The figure shows three views and two pictorial views of one solid part (mm, origin at its lowest corner). Answer the questions. A direction names the side the tool comes from. Give positions to 0.01 mm unless a question says otherwise; leave off trailing zeros. Loops run counter-clockwise (first coordinate to the right, second up) from the corner with the lowest first, then second, coordinate; pieces in that order, holes last. Notation, with made-up numbers: (6.25, 4) - (50.25, 4) arc R24 ccw to (50.25, 16) - close; hole circle Ø3 at (43, 65). An arc over 180 degrees is marked (long way). Write each question's results on one line, items separated by ' | '.
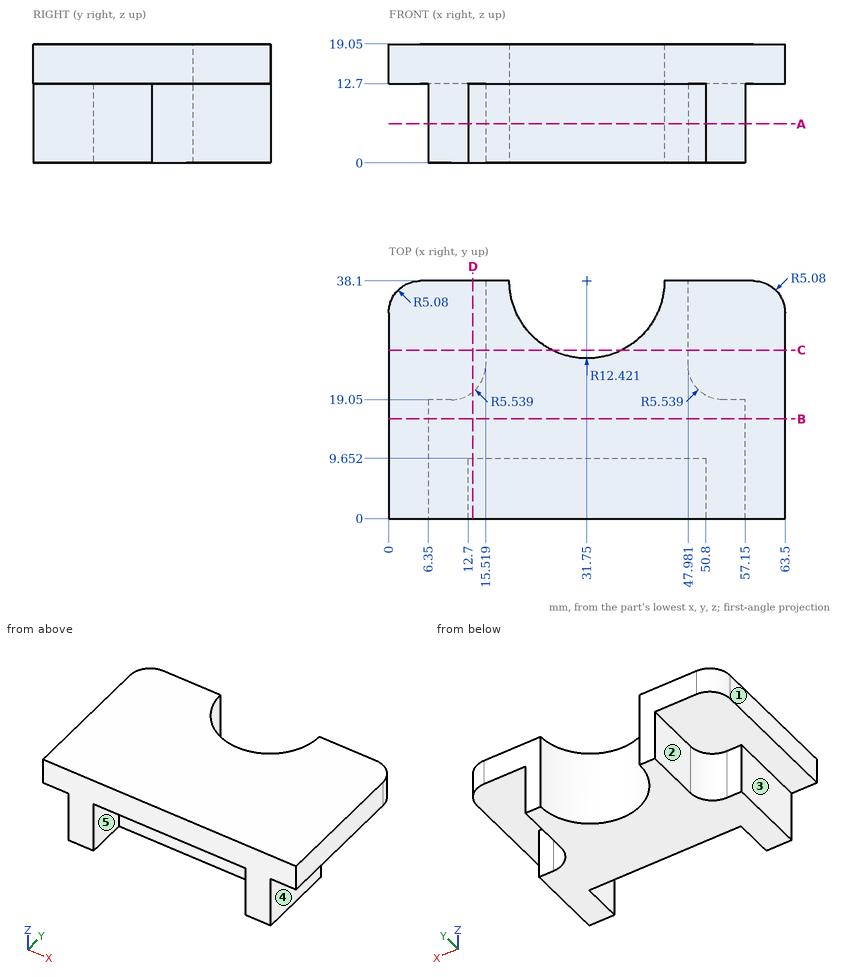
Item 1: A cutting plane is placed at B-B, the plane y = 16. Determine the outline of the cut face in (x, z), plus the area to 3 significant figures.
Values found:
outline: (0, 12.7) - (6.35, 12.7) - (6.35, 0) - (57.15, 0) - (57.15, 12.7) - (63.5, 12.7) - (63.5, 19.05) - (0, 19.05) - close | area: 1,050 mm²
Item 2: Find the intervals of material crossed by line 1 along X through (y, z) = (9.5, 11.5); line 2 along X through (y, z) = (15.5, 3.5); line 3 along Z through (x, y) = (4, 26), in increasing order. Write a range as [from, to].
Values found:
line 1: x = [6.35, 12.7], [50.8, 57.15] | line 2: x = [6.35, 57.15] | line 3: z = [12.7, 19.05]
Item 3: Flat-ended cylindrical pins translate along their axes: P1, Ø4, axis at x = 8.5, z = 7, coming from the +Y side; P2, Ø5, axis at x = 38, y = 5.5, coming from the -Z side; P3, Ø5, axis at y = 4, z = 3.5, coming from the -X side. Find the tip coordinate at first contact, or state that the pin passes through.
Values found:
P1: stops at y = 19.07 | P2: stops at z = 12.7 | P3: stops at x = 6.35
Item 4: A cutting plane is placed at A-A, the plane z = 6.25. Determine the outline of the cut face in (x, y).
Values found:
outline: (6.35, 0) - (12.7, 0) - (12.7, 9.65) - (50.8, 9.65) - (50.8, 0) - (57.15, 0) - (57.15, 19.05) - (53.52, 19.05) arc R5.54 cw to (47.98, 24.59) - (47.98, 38.1) - (44.17, 38.1) arc R12.42 cw to (19.33, 38.1) - (15.52, 38.1) - (15.52, 24.59) arc R5.54 cw to (9.98, 19.05) - (6.35, 19.05) - close
Item 5: A cutting plane is placed at C-C, the plane y = 27. Determine the outline of the cut face in (x, z).
Values found:
outline: (0, 12.7) - (15.52, 12.7) - (15.52, 0) - (26.18, 0) - (26.18, 19.05) - (0, 19.05) - close; (37.32, 0) - (47.98, 0) - (47.98, 12.7) - (63.5, 12.7) - (63.5, 19.05) - (37.32, 19.05) - close
Item 6: A cutting plane is placed at D-D, the plane x = 13.5. Determine the outline of the cut face in (y, z), plus the area to 3 significant figures.
Values found:
outline: (0, 12.7) - (9.65, 12.7) - (9.65, 0) - (20.31, 0) - (20.31, 12.7) - (38.1, 12.7) - (38.1, 19.05) - (0, 19.05) - close | area: 377 mm²
Item 7: For the marked faces 1, 2, 3, 4 and 5, determine the directions among +Z, -Z, +X, -X, +Y, -Y from which every point of the face is accessible in a straight line to the end or side of a thin tool.
Values found:
face 1: +Z, -Z, -X, +Y, -Y | face 2: -Z, -X, +Y | face 3: -Z, -X, +Y, -Y | face 4: -Z, +X, +Y, -Y | face 5: -Z, -Y
